```python
from build123d import *

# Parameters (mm, degrees)
CUT_EXTRUDE_1_DEPTH = 10
SKETCH_4_R          = 2.65
CUT_EXTRUDE_2_DEPTH = 5


with BuildPart() as part:
    # 草图2 → 旋转1 (revolve)
    with BuildSketch(Plane(origin=(0, 0, 0), x_dir=(1, 0, 0), z_dir=(0, 1, 0))):
        with BuildLine():
            Line((0, 0), (0, 28))
            Line((0, 28), (30, 28))
            ThreePointArc((30, 28), (34, 15.5), (30, 3))
            Line((30, 3), (4.85, 3))
            Line((4.85, 3), (4.85, 0))
            Line((4.85, 0), (0, 0))
        make_face()
    revolve(axis=Axis((0, 0, 0), (0, 0, -1)))

    # 草图3 → 切除-拉伸1 (cut)
    with BuildSketch(Plane.XY):
        with BuildLine():
            Line((1.989974874, 1.75), (-1.989974874, 1.75))
            ThreePointArc((-1.989974874, 1.75), (-2.65, 0), (-1.989974874, -1.75))
            Line((-1.989974874, -1.75), (1.989974874, -1.75))
            ThreePointArc((1.989974874, -1.75), (2.65, 0), (1.989974874, 1.75))
        make_face()
    extrude(amount=-CUT_EXTRUDE_1_DEPTH, mode=Mode.SUBTRACT)

    # 草图4 → 切除-拉伸2 (cut)
    with BuildSketch(Plane.XY):
        Circle(SKETCH_4_R)
    extrude(amount=-CUT_EXTRUDE_2_DEPTH, mode=Mode.SUBTRACT)


solid = part.part
```
Geometry: final body of the model. Coordinates: model frame, mm. A direction names the side the tool comes from. Coordinates: 2 decimals unless noted, no trailing zeros. Order: outer loops, then holes, each group sorted by start corner. A loop starts at its lowest first (then second) coordinate and runs counter-clockwise, first axis right, second up. Notation, with made-up numbers: (-39.5, 31) - (6.5, 31) arc R25 ccw to (6.5, 60) - close; hole circle Ø7 at (46.5, 20.25). An arc over 180 degrees is marked (long way). Write each question's results on one line, items separated by ' | '.
1) Pin query (flat end, axial travel): pin 1 (12 mm diameter, centred on x = -21.5, z = -15.5, fed in from -Y); pin 2 (5 mm diameter, centred on x = -8.5, z = -6.5, fed in from +Y); pin 3 (2 mm diameter, centred on x = -0.5, z = -8, fed in from -Y). Return the tip coordinate at first contact, or that it passes through.
Results list:
pin 1: y = -30.26 | pin 2: y = 32.08 | pin 3: y = -32.99
2) Pull-direction query (Y, two-part tool) for faces 3 (the flat face through (2, 2, 0)), 4 (the flat face through (0, -1.75, -7)), 5 (the cylindrical face through (4.626, -1.457, -1.479)); classes: pulls with the +Y half, pulls with the -Y half, needs draft (parallel to the pull), parting line crosses it, or undercut.
Results list:
face 3: needs draft | face 4: undercut | face 5: parting line crosses it
3) Section A-A, the plane z = -2. Return loops of the section in (x, y).
Results list:
outline: circle Ø9.7 at (0, 0); hole circle Ø5.3 at (0, 0)
4) Set-up query: faces 1 (the flat face through (0, 1.75, -7)), 2 (the flat face through (0, 0, -28)). Return all of +Z, -Z, +X, -X, +Y, -Y with unobstructed straight access to the full face (end or side cutting, diameter ignored); none if empty.
Results list:
face 1: +Z | face 2: -Z, +X, -X, +Y, -Y
5) Line query: line 1 (Z direction, x = -3, y = -20.5); line 2 (X direction, y = 0, z = -5.25); line 3 (X direction, y = -1.5, z = -6.5). Output: solid intervals per line, ascending. Write a range as from..to.
Results list:
line 1: -28..-3 | line 2: -31.4..-2.65, 2.65..31.4 | line 3: -31.99..-2.18, 2.18..31.99
